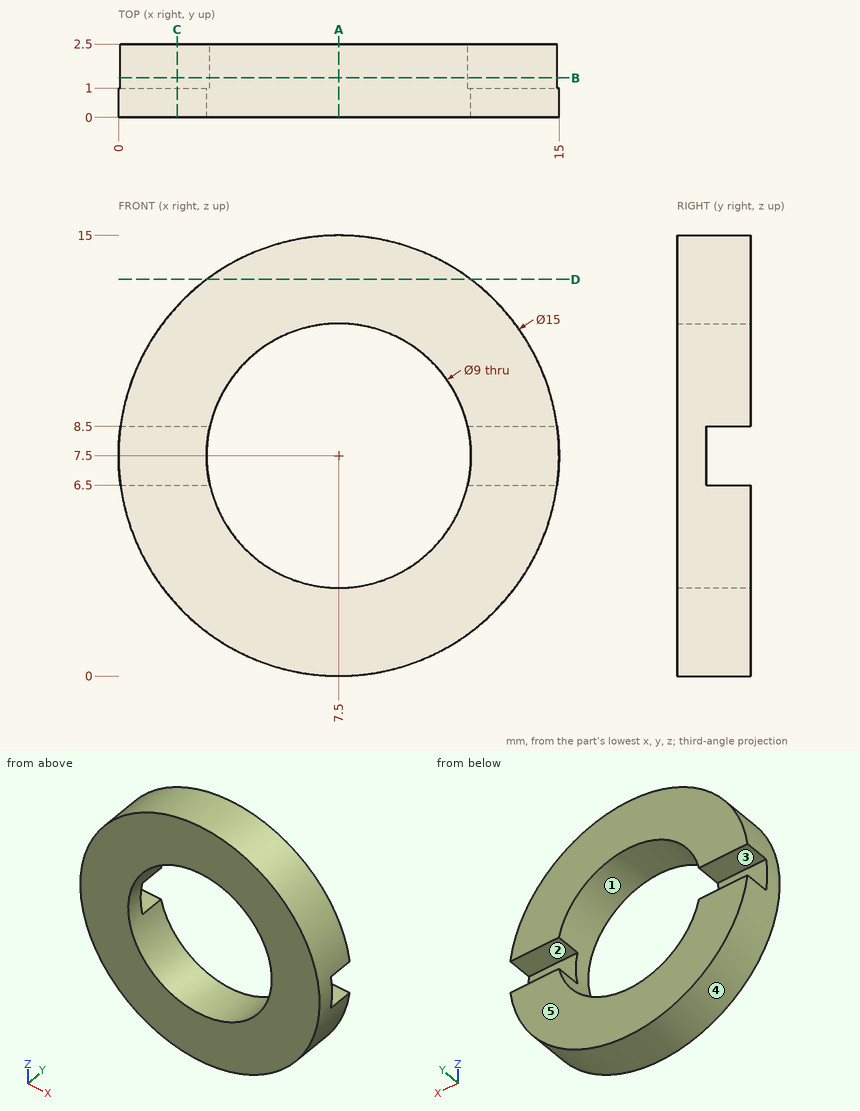
The drawing under review shows one solid part. Ordinate dimensions are in mm from its lowest x, y, z. A direction names the side the tool comes from. Give positions to 0.01 mm unless a question says otherwise; leave off trailing zeros. Write each loop counter-clockwise with the first axis right and the second up, starting at its lowest first coordinate (ties: lowest second). Pieces come first, ordered by that corner, then holes.
1. Wall thickness on L1, parallel to Z at x = 6.5, y = 0.95; L2, parallel to Z at x = 13.5, y = 1.55; L3, parallel to X at y = 1.45, z = 10: over which ranges is each line inside the solid? List them lowest first.
2. Draft analysis for pull direction Z (two halves, no side actions). For the marked faces 3, 4 and 5, state which applies: +Z half, -Z half, draft (parallel to the pull), parting line (faces both ways), or undercut.
3. Add section B-B, the plane y = 1.35. Write out the cut boundary in (x, z).
4. Add section A-A, the plane x = 7.5. Write out the cut boundary in (y, z), plus the area to 3 significant figures.
5. Tool access review of the marked faces 1 and 2: name each direction out of +Z, -Z, +X, -X, +Y, -Y from which nothing blocks a thin tool from reaching the whole face with its end or side.
6. Add section D-D, the plane z = 13.5. Write out the cut boundary in (x, y), plus the area to 3 significant figures.
7. Add section C-C, the plane x = 2. Write out the cut boundary in (y, z), plus the area to 3 significant figures.
8. For P1, Ø1.6, axis at x = 1.5, z = 7.5, coming from the +Y side; P2, Ø1.2, axis at x = 2, y = 2, coming from the -Z side; P3, Ø0.8, axis at x = 14, y = 1.5, coming from the -Z side, all flat-tipped, find the tip position at first contact; note any pin that passes through.
Worked answers:
1. L1: z = 0.07 to 3.11, 11.89 to 14.93
1. L2: z = 3 to 6.5, 8.5 to 12
1. L3: x = 0.43 to 3.76, 11.24 to 14.57
2. face 3: undercut
2. face 4: parting line
2. face 5: draft
3. outline: (0.07, 6.5) arc R7.5 ccw to (14.93, 6.5) - (11.89, 6.5) arc R4.5 cw to (3.11, 6.5) - close; (0.07, 8.5) - (3.11, 8.5) arc R4.5 cw to (11.89, 8.5) - (14.93, 8.5) arc R7.5 ccw to start
4. outline: (0, 0) - (2.5, 0) - (2.5, 3) - (0, 3) - close; (0, 12) - (2.5, 12) - (2.5, 15) - (0, 15) - close
4. area: 15.0 mm2
5. face 1: +Y, -Y
5. face 2: +X, -X, +Y
6. outline: (3, 0) - (12, 0) - (12, 2.5) - (3, 2.5) - close
6. area: 22.5 mm2
7. outline: (0, 2.4) - (2.5, 2.4) - (2.5, 6.5) - (1, 6.5) - (1, 8.5) - (2.5, 8.5) - (2.5, 12.6) - (0, 12.6) - close
7. area: 22.5 mm2
8. P1: stops at y = 1
8. P2: stops at z = 1.82
8. P3: stops at z = 3.14
